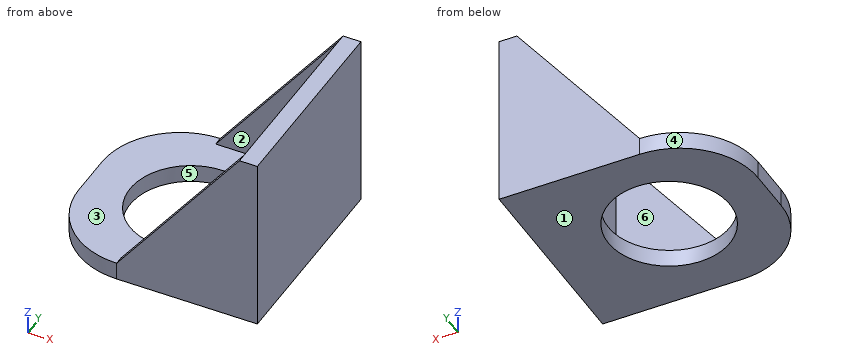
from build123d import *

# Parameters (mm, degrees)
SKETCH_W     = 45
SKETCH_H     = 45
SKETCH_R     = 13.6
PAD_DEPTH    = 4
SKETCH001_W  = 45
SKETCH001_H  = 40
PAD001_DEPTH = 4
FILLET_R     = 17.5
PAD002_DEPTH = 2


with BuildPart() as part:
    # Sketch → Pad (new body)
    with BuildSketch(Plane.XY):
        Rectangle(SKETCH_W, SKETCH_H)
        Circle(SKETCH_R, mode=Mode.SUBTRACT)
    extrude(amount=PAD_DEPTH)

    # Sketch001 (on Face3 of Pad) → Pad001 (join)
    with BuildSketch(Plane.YZ.offset(22.5)):
        with Locations((0, 20)):
            Rectangle(SKETCH001_W, SKETCH001_H)
    extrude(amount=PAD001_DEPTH)

    # Fillet
    fillet_edges = [part.edges().sort_by_distance(p)[0] for p in [
        (-22.5, 22.5, 2),
        (-22.5, -22.5, 2),
    ]]
    fillet(fillet_edges, radius=FILLET_R)

    # Sketch002 (on Face6 of Fillet) → Pad002 (join)
    with BuildSketch(Plane.XZ.offset(22.5)):
        Polygon((-5, 4), (22.5, 4), (22.5, 40), align=None)
    pad002 = extrude(amount=-PAD002_DEPTH)

    # Mirrored: Pad002 across XZ
    add(pad002.mirror(Plane.XZ))


solid = part.part
Work out the finished part from the listing and answer in its coordinate system (mm). Face numbers are marked on the shaded views. A direction names the side the tool comes from. Round coordinates to 2 decimals unless told otherwise and drop trailing zeros. Write each loop counter-clockwise with the first axis right and the second up, starting at its lowest first coordinate (ties: lowest second). Pieces come first, ordered by that corner, then holes. Notation, with made-up numbers: M -27,-34.75 L -23,-34.75 A33 cw -23,-2.75 Z; hole C 1,86 d1. An arc over 180 degrees is marked long. Use a Markdown table: item, result.
1) The part is cut by section C-C on z = 6.5. Give the vertices of the cut face in (x, y), plus the area to 3 significant figures.
Taken from the geometry:
| item | result |
|---|---|
| outline | M -3.09,-22.5 L 26.5,-22.5 L 26.5,22.5 L -3.09,22.5 L -3.09,20.5 L 22.5,20.5 L 22.5,-20.5 L -3.09,-20.5 Z |
| area | 282 mm2 |
2) Consider line 1 (Y direction, x = 5, z = 14); line 2 (Y direction, x = 0, z = 2); line 3 (Z direction, x = 13, y = -13.5). Determine where each line is inside the solid, lowest interval first. Write a range as [from, to].
Taken from the geometry:
| item | result |
|---|---|
| line 1 | y = [-22.5, -20.5], [20.5, 22.5] |
| line 2 | y = [-22.5, -13.6], [13.6, 22.5] |
| line 3 | z = [0, 4] |
3) The part is cut by section B-B on x = 0. Give the vertices of the cut face in (y, z), plus the area to 3 significant figures.
Taken from the geometry:
| item | result |
|---|---|
| outline | M -22.5,0 L -13.6,0 L -13.6,4 L -20.5,4 L -20.5,10.55 L -22.5,10.55 Z; M 13.6,0 L 22.5,0 L 22.5,10.55 L 20.5,10.55 L 20.5,4 L 13.6,4 Z |
| area | 97.4 mm2 |
4) The part is cut by section D-D on x = -8. Give the vertices of the cut face in (y, z).
Taken from the geometry:
| item | result |
|---|---|
| outline | M -22.24,0 L -11,0 L -11,4 L -22.24,4 Z; M 11,0 L 22.24,0 L 22.24,4 L 11,4 Z |
5) Which of the six approach directions +Z, -Z, +X, -X, +Y, -Y give full straight-line access (tool end or side, diameter ignored) to the marked faces 5 and 6?
Taken from the geometry:
| item | result |
|---|---|
| face 5 | +Z, -Z |
| face 6 | +Z, -X |
6) The part is cut by section A-A on y = 0. Give the vertices of the cut face in (x, z), plus the area to 3 significant figures.
Taken from the geometry:
| item | result |
|---|---|
| outline | M -22.5,0 L -13.6,0 L -13.6,4 L -22.5,4 Z; M 13.6,0 L 26.5,0 L 26.5,40 L 22.5,40 L 22.5,4 L 13.6,4 Z |
| area | 231 mm2 |
7) Flat-ended cylindrical pins translate along their axes: pin 1 (5 mm diameter, centred on y = -13, z = 6, fed in from -X); pin 2 (10 mm diameter, centred on y = 13.5, z = 27.5, fed in from -X). Find the tip coordinate at first contact, or state that the pin passes through.
Taken from the geometry:
| item | result |
|---|---|
| pin 1 | stops at x = -21.25 |
| pin 2 | stops at x = 22.5 |
8) Determine the mould class of the marked faces 1, 2, 3 and 4 for opening direction Y: pulls with the +Y half, pulls with the -Y half, needs draft (parallel to the pull), parting line crosses it, or undercut.
Taken from the geometry:
| item | result |
|---|---|
| face 1 | needs draft |
| face 2 | undercut |
| face 3 | undercut |
| face 4 | pulls with the +Y half |
